Verification items for the finished model (mm, model axes). A direction names the side the tool comes from. Coordinates: 2 decimals unless noted, no trailing zeros. Order: outer loops, then holes, each group sorted by start corner. A loop starts at its lowest first (then second) coordinate and runs counter-clockwise, first axis right, second up. Notation, with made-up numbers: M 39.25,0.25 L 74.25,0.25 A19 cw 74.25,23.25 Z; hole C 17,-5.5 d9. An arc over 180 degrees is marked long. Answer as a JSON object with one key per item and string values. Group by question number.
(1) Gauge pin test, flat ends, axial feed: pin 1 Ø12 at (y, z) = (0, 70) entering from +X; pin 2 Ø1.8 at (x, y) = (-55, 7) entering from -Z; pin 3 Ø4 at (x, y) = (37, -4) entering from -Z; pin 4 Ø5 at (x, y) = (55, -7) entering from +Z. Record the tip position at first contact, or that the pin passes through.
(2) Cross-section at A-A (z = 8.5). Enter the section's corners in (x, y), plus the area to 3 significant figures.
(3) Cross-section at C-C (z = 19). Enter the section's corners in (x, y), plus the area to 3 significant figures.
(4) Cross-section at D-D (x = -55). Enter the section's corners in (y, z).
(5) Material ranges on line 1 (Y direction, x = 55, z = 4); line 2 (X direction, y = 3.75, z = 45.5); line 3 (Z direction, x = -49, y = -0.25), recorded low to high.
(6) Access from +Z, -Z, +X, -X, +Y, -Y to the whole of each face (thin tool, end or side, straight path). Record for faces 1 (the face through (-60, 0, 33)), 2 (the face through (-55, 7, 15)), 3 (the face through (0.812, 0.66, 84.985)).
(7) Mould release check, pull along Y, two halves, no side actions. Record for faces 4 (the face through (60, 0, 32)), 5 (the face through (-56.386, 6.425, 7.395)), 6 (the face through (-54, -15, 35)): released by +Y, released by -Y, zero draft, split by the parting line, or undercut.
(8) Cross-section at B-B (y = 0). Enter the section's corners in (x, z), plus the area to 3 significant figures.
from build123d import *

# Parameters (mm, degrees)
SKETCH1_W                      = 10
SKETCH1_H                      = 30
BOSS_EXTRUDE1_DEPTH            = 70
BOSS_EXTRUDE1_2_DEPTH          = 70
SKETCH2_R                      = 15
BOSS_EXTRUDE2_DEPTH            = 120
CUT_EXTRUDE1_REACH             = 122
SKETCH3_R                      = 10
CUT_EXTRUDE1_DIRECTION_2_DEPTH = 1
FILLET1_R                      = 2
SKETCH4_R                      = 1.5
CUT_EXTRUDE2_DEPTH             = 15


with BuildPart() as part:
    # Sketch1 → Boss-Extrude1 (new body)
    with BuildSketch(Plane.XY):
        with Locations((55, 0)):
            Rectangle(SKETCH1_W, SKETCH1_H)
    extrude(amount=BOSS_EXTRUDE1_DEPTH)



with BuildPart() as body_2:
    # Sketch1 → Boss-Extrude1 2 (new body)
    with BuildSketch(Plane.XY):
        with Locations((-55, 0)):
            Rectangle(SKETCH1_W, SKETCH1_H)
    extrude(amount=BOSS_EXTRUDE1_2_DEPTH)


with BuildPart() as part_1:
    add(part.part)

    add(body_2.part)  # Boss-Extrude2 merges body 2
    # Sketch2 → Boss-Extrude2 (add)
    with BuildSketch(Plane(origin=(60, 0, 0), x_dir=(0, 0, -1), z_dir=(1, 0, 0))):
        with Locations((-70, 0)):
            Circle(SKETCH2_R)
    extrude(amount=-BOSS_EXTRUDE2_DEPTH)

    # Sketch3 → Cut-Extrude1 (cut, up to next)
    with BuildSketch(Plane.ZY.offset(60), mode=Mode.PRIVATE) as cut_extrude1_sk1:
        with Locations((70, 0)):
            Circle(SKETCH3_R)
    cut_extrude1_tool1 = extrude(cut_extrude1_sk1.sketch, amount=-CUT_EXTRUDE1_REACH, mode=Mode.PRIVATE) & part_1.part
    add(cut_extrude1_tool1.solids().sort_by_distance((-60, 0, 70))[0], mode=Mode.SUBTRACT)

    # Sketch3 → Cut-Extrude1 direction 2 (cut)
    with BuildSketch(Plane.ZY.offset(60)):
        with Locations((70, 0)):
            Circle(SKETCH3_R)
    extrude(amount=CUT_EXTRUDE1_DIRECTION_2_DEPTH, mode=Mode.SUBTRACT)

    # Fillet1
    fillet1_edges = [part_1.edges().sort_by_distance(p)[0] for p in [
        (60, 0, 85),
        (-60, 0, 85),
        (-60, 15, 35),
        (-60, -15, 35),
        (-60, 0, 60),
        (60, 0, 60),
        (60, 15, 35),
        (60, -15, 35),
    ]]
    fillet(fillet1_edges, radius=FILLET1_R)

    # Sketch4 → Cut-Extrude2 (cut)
    with BuildSketch(Plane(origin=(0, 0, 0), x_dir=(-1, 0, 0), z_dir=(0, 0, -1))):
        with Locations((-55, 7)):
            Circle(SKETCH4_R)
        with Locations((-55, -7)):
            Circle(SKETCH4_R)
        with Locations((55, -7)):
            Circle(SKETCH4_R)
        with Locations((55, 7)):
            Circle(SKETCH4_R)
    extrude(amount=-CUT_EXTRUDE2_DEPTH, mode=Mode.SUBTRACT)


solid = part_1.part
Taken from the geometry:
{
 "1": {"pin 1": "passes through", "pin 2": "stops at z = 15", "pin 3": "stops at z = 55.13", "pin 4": "stops at z = 84.31"},
 "2": {"outline": "M -60,-13 A2 ccw -58,-15 L -50,-15 L -50,15 L -58,15 A2 ccw -60,13 Z; M 50,-15 L 58,-15 A2 ccw 60,-13 L 60,13 A2 ccw 58,15 L 50,15 Z; hole C -55,-7 d3; hole C -55,7 d3; hole C 55,-7 d3; hole C 55,7 d3", "area": "568 mm²"},
 "3": {"outline": "M -60,-13 A2 ccw -58,-15 L -50,-15 L -50,15 L -58,15 A2 ccw -60,13 Z; M 50,-15 L 58,-15 A2 ccw 60,-13 L 60,13 A2 ccw 58,15 L 50,15 Z", "area": "597 mm²"},
 "4": {"outline": "M -15,0 L -8.5,0 L -8.5,15 L -5.5,15 L -5.5,0 L 5.5,0 L 5.5,15 L 8.5,15 L 8.5,0 L 15,0 L 15,70 A15 ccw -15,70 Z; hole C 0,70 d20"},
 "5": {"line 1": "y = -15 to -8.5, -5.5 to 5.5, 8.5 to 15", "line 2": "x = -60 to -50, 50 to 60", "line 3": "z = 55 to 60, 80 to 85"},
 "6": {"face 1": "+Z, -Z, -X, +Y, -Y", "face 2": "-Z", "face 3": "none"},
 "7": {"face 4": "zero draft", "face 5": "undercut", "face 6": "released by -Y"},
 "8": {"outline": "M -60,0 L -50,0 L -50,55 L 50,55 L 50,0 L 60,0 L 60,58 A2 ccw 58,60 L -58,60 A2 ccw -60,58 Z; M -60,82 A2 ccw -58,80 L 58,80 A2 ccw 60,82 L 60,83 A2 ccw 58,85 L -58,85 A2 ccw -60,83 Z", "area": "2,290 mm²"}
}
